from build123d import *

# Parameters (mm, degrees)
F0_R     = 1.9
F1_DEPTH = 3
F2_W     = 25.4
F2_H     = 25.4
F2_W_2   = 19.4
F2_H_2   = 19.4
F3_DEPTH = 12.7


with BuildPart() as f1:
    # F0 (on Top) → F1 (new body)
    with BuildSketch(Plane.XY):
        Polygon((-19.25, 19.25), (-19.25, 0), (-19.25, -19.25), (19.25, -19.25), (19.25, 19.25), align=None)
        with Locations((-15.95, -15.95)):
            Circle(F0_R, mode=Mode.SUBTRACT)
        with Locations((15.95, -15.95)):
            Circle(F0_R, mode=Mode.SUBTRACT)
        with Locations((-15.95, 15.95)):
            Circle(F0_R, mode=Mode.SUBTRACT)
        with Locations((15.95, 15.95)):
            Circle(F0_R, mode=Mode.SUBTRACT)
    extrude(amount=F1_DEPTH)

    # F2 (on face) → F3 (join)
    with BuildSketch(Plane.XY.offset(3)):
        Rectangle(F2_W, F2_H)
        Rectangle(F2_W_2, F2_H_2, mode=Mode.SUBTRACT)
    extrude(amount=F3_DEPTH)


solid = f1.part
Input: part model. Units: mm. Frame: model coordinates. A direction names the side the tool comes from. Give positions to 0.01 mm unless a question says otherwise; leave off trailing zeros. Order: outer loops, then holes, each group sorted by start corner. A loop starts at its lowest first (then second) coordinate and runs counter-clockwise, first axis right, second up.
Q1. Section B-B on z = 13.25. Output: boundary loops of the cut face in (x, y), and give its area (3 significant figures).
Checked values:
outline: (-12.7, -12.7) - (12.7, -12.7) - (12.7, 12.7) - (-12.7, 12.7) - close; hole (-9.7, -9.7) - (9.7, -9.7) - (9.7, 9.7) - (-9.7, 9.7) - close
area: 269 mm2
Q2. Section A-A on y = 15.95. Output: boundary loops of the cut face in (x, z).
Checked values:
outline: (-19.25, 0) - (-17.85, 0) - (-17.85, 3) - (-19.25, 3) - close; (-14.05, 0) - (14.05, 0) - (14.05, 3) - (-14.05, 3) - close; (17.85, 0) - (19.25, 0) - (19.25, 3) - (17.85, 3) - close
Q3. Set-up query: faces 1 (the flat face through (0, 12.7, 9)), 2 (the flat face through (0, 0, 3)), 3 (the flat face through (12.7, 0, 9)). Return all of +Z, -Z, +X, -X, +Y, -Y with unobstructed straight access to the full face (end or side cutting, diameter ignored); none if empty.
Checked values:
face 1: +Z, +X, -X, +Y
face 2: +Z
face 3: +Z, +X, +Y, -Y
Q4. Contact query for flat-ended pins moving along their axis: pin 1 Ø4 at (x, z) = (4, 9.5) entering from +Y; pin 2 Ø6.5 at (y, z) = (-0.5, 12.5) entering from +X; pin 3 Ø4 at (x, z) = (-3.5, 9) entering from -Y. Output: stop coordinate, or through.
Checked values:
pin 1: stops at y = 12.7
pin 2: stops at x = 12.7
pin 3: stops at y = -12.7
Q5. Draft query along X for faces 4 (the flat face through (0, -9.7, 9)), 5 (the flat face through (0, 19.25, 1)), 6 (the flat face through (-12.7, 0, 9)), 7 (the flat face through (9.7, 0, 9)). Return one class per face: +X half, -X half, draft (parallel to the pull), parting line (faces both ways), or undercut.
Checked values:
face 4: undercut
face 5: draft
face 6: -X half
face 7: undercut
Q6. Section D-D on x = 12. Output: boundary loops of the cut face in (y, z).
Checked values:
outline: (-19.25, 0) - (19.25, 0) - (19.25, 3) - (12.7, 3) - (12.7, 15.7) - (-12.7, 15.7) - (-12.7, 3) - (-19.25, 3) - close
Q7. Ray query, probe 1 along Y at (x, z) = (-15.95, 2.1); probe 2 along Y at (x, z) = (-8.5, 7). Return the intervals inside material, ascending.
Checked values:
probe 1: y = -19.25 to -17.85, -14.05 to 14.05, 17.85 to 19.25
probe 2: y = -12.7 to -9.7, 9.7 to 12.7
